The model under review builds one solid part; all positions refer to its coordinate system, in mm. A direction names the side the tool comes from. Give positions to 0.01 mm unless a question says otherwise; leave off trailing zeros. Loops run counter-clockwise (first coordinate to the right, second up) from the corner with the lowest first, then second, coordinate; pieces in that order, holes last. Notation, with made-up numbers: M -30,74 L 17,74 A28 ccw 17,96 Z; hole C -19,39 d1. An arc over 180 degrees is marked long. One line per item, written item: value. Start each with the question number.
Q1. We need section A-A on y = -34. Write out the cut boundary in (x, z), plus the area to 3 significant figures.
Q2. For faces 1 (the face through (-16, -19, -4.353)), 2 (the face through (-17, -30, -2.353)), 3 (the face through (4, -18, -3)), list the 3-axis set-ups (+Z, -Z, +X, -X, +Y, -Y) from which the entire face can be reached by the end or side of a thin tool; tool diameter is ignored.
Q3. We need section D-D on x = -1. Write out the cut boundary in (y, z), plus the area to 3 significant figures.
Q4. To check wall thickness, follow line 1 along X through (y, z) = (-6, -3); line 2 along X through (y, z) = (-5, -5); line 3 along X through (y, z) = (-8.5, -5.75). State the ranges of each line that lie inside material, in increasing order. Write a range as from..to.
Q5. We need section C-C on y = -7. Write out the cut boundary in (x, z).
Q6. Mouldability with a two-part tool opening along Y and no side actions: class faces 4 (the face through (16, -14.382, -3)), 5 (the face through (-8, -18, -3)) as released by +Y, released by -Y, zero draft, split by the parting line, or undercut.
Q7. For pin 1 (2 mm diameter, centred on x = -17.5, y = -17, fed in from -Z); pin 2 (4.5 mm diameter, centred on x = -17, z = -4, fed in from -Y); pin 3 (3 mm diameter, centred on x = 15.5, y = -31, fed in from -Z); pin 4 (1.9 mm diameter, centred on x = 16, z = -2.5, fed in from +Y), all flat-tipped, find the tip position at first contact; note any pin that passes through.
Q8. We need section B-B on x = -14.5. Write out the cut boundary in (y, z).
```python
from build123d import *

# Parameters (mm, degrees)
F0_W     = 4
F0_H     = 4
F0_W_2   = 2
F0_H_2   = 2
F1_DEPTH = 36
F2_W     = 4
F2_H     = 4
F2_W_2   = 2
F2_H_2   = 2
F3_DEPTH = 4
F4_W     = 4
F4_H     = 4
F4_W_2   = 2
F4_H_2   = 2
F5_DEPTH = 4


with BuildPart() as f1:
    # F0 (on Front) → F1 (new body)
    with BuildSketch(Plane.XZ):
        Polygon((16, -2), (18, -2), (18, 2), (-18, 2), (-18, -2), (-16, -2), (-10, -2), (-8, -2), (-6, -2), (-2, -2), (0, -2), (2, -2), (4, -2), (8, -2), (12, -2), align=None)
        with Locations((10, -4)):
            Rectangle(F0_W, F0_H)
        with Locations((3, -3)):
            Rectangle(F0_W_2, F0_H_2)
        Polygon((-10, -2), (-16, -2), (-16, -4), (-12, -4), (-12, -6), (-10, -6), align=None)
        with Locations((-1, -4)):
            Rectangle(F0_W_2, F0_H)
        with Locations((-7, -3)):
            Rectangle(F0_W_2, F0_H_2)
    extrude(amount=F1_DEPTH)

    # F2 (on face) → F3 (join)
    with BuildSketch(Plane.YZ.offset(18)):
        with Locations((-6.381626, -3.717597)):
            Rectangle(F2_W, F2_H)
        Polygon((-26.381626, -5.717597), (-26.381626, -1.717597), (-32.381626, -1.717597), (-32.381626, -3.717597), (-28.381626, -3.717597), (-28.381626, -5.717597), align=None)
        with Locations((-23.381626, -2.717597)):
            Rectangle(F2_W_2, F2_H_2)
        with Locations((-17.381626, -3.717597)):
            Rectangle(F2_W_2, F2_H)
        with Locations((-13.381626, -2.717597)):
            Rectangle(F2_W_2, F2_H_2)
    extrude(amount=-F3_DEPTH)

    # F4 (on face) → F5 (join)
    with BuildSketch(Plane(origin=(-18, 0, 0), x_dir=(0, -1, 0), z_dir=(-1, 0, 0))):
        Polygon((27.795796, -2.352679), (31.795796, -2.352679), (31.795796, 1.647321), (-0.204204, 1.647321), (-0.204204, -2.352679), (5.795796, -2.352679), (7.795796, -2.352679), (9.795796, -2.352679), (13.795796, -2.352679), (15.795796, -2.352679), (17.795796, -2.352679), (19.795796, -2.352679), (23.795796, -2.352679), align=None)
        with Locations((25.795796, -4.352679)):
            Rectangle(F4_W, F4_H)
        with Locations((18.795796, -3.352679)):
            Rectangle(F4_W_2, F4_H_2)
        Polygon((5.795796, -2.352679), (-0.204204, -2.352679), (-0.204204, -4.352679), (3.795796, -4.352679), (3.795796, -6.352679), (5.795796, -6.352679), align=None)
        with Locations((14.795796, -4.352679)):
            Rectangle(F4_W_2, F4_H)
        with Locations((8.795796, -3.352679)):
            Rectangle(F4_W_2, F4_H_2)
    extrude(amount=-F5_DEPTH)


solid = f1.part
```
Solved:
1. outline: M -18,-2 L -16,-2 L -16,-4 L -12,-4 L -12,-6 L -10,-6 L -10,-2 L -8,-2 L -8,-4 L -6,-4 L -6,-2 L -2,-2 L -2,-6 L 0,-6 L 0,-2 L 2,-2 L 2,-4 L 4,-4 L 4,-2 L 8,-2 L 8,-6 L 12,-6 L 12,-2 L 18,-2 L 18,2 L -18,2 Z
1. area: 192 mm2
2. face 1: -Z, -X
2. face 2: -Z, -X, -Y
2. face 3: -Z, +Y, -Y
3. outline: M -36,-6 L 0,-6 L 0,2 L -36,2 Z
3. area: 288 mm2
4. line 1: -16..-10, -8..-6, -2..0, 2..4, 8..12, 14..18
4. line 2: -18..-14, -12..-10, -2..0, 8..12, 14..18
4. line 3: -12..-10, -2..0, 8..12
5. outline: M -18,-2.35 L -16,-2.35 L -16,-4 L -12,-4 L -12,-6 L -10,-6 L -10,-2 L -8,-2 L -8,-4 L -6,-4 L -6,-2 L -2,-2 L -2,-6 L 0,-6 L 0,-2 L 2,-2 L 2,-4 L 4,-4 L 4,-2 L 8,-2 L 8,-6 L 12,-6 L 12,-2 L 14,-2 L 14,-5.72 L 18,-5.72 L 18,2 L -18,2 Z
6. face 4: undercut
6. face 5: zero draft
7. pin 1: z = -4.35
7. pin 2: y = -36
7. pin 3: z = -3.72
7. pin 4: y = 0
8. outline: M -36,-4 L -27.8,-4 L -27.8,-6.35 L -23.8,-6.35 L -23.8,-4 L -19.8,-4 L -19.8,-4.35 L -17.8,-4.35 L -17.8,-4 L -15.8,-4 L -15.8,-6.35 L -13.8,-6.35 L -13.8,-4 L -9.8,-4 L -9.8,-4.35 L -7.8,-4.35 L -7.8,-4 L -5.8,-4 L -5.8,-6.35 L -3.8,-6.35 L -3.8,-4.35 L 0.2,-4.35 L 0.2,1.65 L 0,1.65 L 0,2 L -36,2 Z
